Design review of the part built by this model. Coordinates are the model's own, in mm. Face numbers are marked on the shaded views. A direction names the side the tool comes from. Coordinates: 2 decimals unless noted, no trailing zeros. Loops run counter-clockwise (first coordinate to the right, second up) from the corner with the lowest first, then second, coordinate; pieces in that order, holes last. Notation, with made-up numbers: M 29,-29.75 L 50,-29.75 A26 cw 50,-1.75 Z; hole C 45.5,79 d11. An arc over 180 degrees is marked long. One line per item, written item: value.
```python
from build123d import *

# Parameters (mm, degrees)
SKETCH1_R           = 3
SKETCH1_R_2         = 1.6
BOSS_EXTRUDE1_DEPTH = 2
SKETCH1_3_R         = 1.6
BOSS_EXTRUDE2_DEPTH = 1
SKETCH5_R           = 1.5
BOSS_EXTRUDE3_DEPTH = 1
SKETCH6_R           = 2
BOSS_EXTRUDE4_DEPTH = 1
SKETCH8_R           = 1
BOSS_EXTRUDE5_DEPTH = 3


with BuildPart() as part:
    # Sketch1 → Boss-Extrude1 (new body)
    with BuildSketch(Plane(origin=(0, 0, 0), x_dir=(1, 0, 0), z_dir=(0, 1, 0))):
        with Locations((-0.522013312, 0.511138034)):
            Circle(SKETCH1_R)
        with Locations((-0.522013312, 0.511138034)):
            Circle(SKETCH1_R_2, mode=Mode.SUBTRACT)
    extrude(amount=BOSS_EXTRUDE1_DEPTH)

    # Sketch1<3> → Boss-Extrude2 (add)
    with BuildSketch(Plane(origin=(0, 0, 0), x_dir=(1, 0, 0), z_dir=(0, 1, 0))):
        with Locations((-0.522013312, 0.511138034)):
            Circle(SKETCH1_3_R)
    extrude(amount=BOSS_EXTRUDE2_DEPTH)

    # Sketch5 → Boss-Extrude3 (add)
    with BuildSketch(Plane.XZ):
        with Locations((-0.522013312, -0.511138034)):
            Circle(SKETCH5_R)
    extrude(amount=BOSS_EXTRUDE3_DEPTH)

    # Sketch6 → Boss-Extrude4 (add)
    with BuildSketch(Plane.XZ.offset(1)):
        with Locations((-0.522013312, -0.511138034)):
            Circle(SKETCH6_R)
    extrude(amount=BOSS_EXTRUDE4_DEPTH)

    # Sketch8 → Boss-Extrude5 (add)
    with BuildSketch(Plane(origin=(0, -2, 0), x_dir=(-1, 0, 0), z_dir=(0, -1, 0))):
        with Locations((0.522013312, 0.511138034)):
            Circle(SKETCH8_R)
    extrude(amount=BOSS_EXTRUDE5_DEPTH)


solid = part.part
```
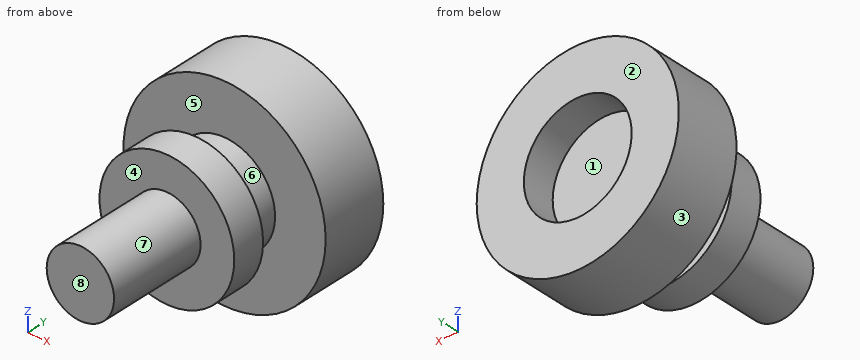
(1) We need section C-C on z = 0.8. State the section outline as (x, y) points (3 decimals), then the cut area to 3 significant figures.
Reply:
outline: M -3.22,0 L -1.251,0 L -1.251,-1 L -2.032,-1 L -2.032,-2 L 0.988,-2 L 0.988,-1 L 0.207,-1 L 0.207,0 L 2.176,0 L 2.176,2 L 0.395,2 L 0.395,1 L -1.439,1 L -1.439,2 L -3.22,2 Z
area: 13.4 mm2
(2) Mouldability with a two-part tool opening along Y and no side actions: class the marked faces 6, 7 and 8 as released by +Y, released by -Y, zero draft, split by the parting line, or undercut.
Reply:
face 6: undercut
face 7: zero draft
face 8: released by -Y
(3) To check wall thickness, follow line 1 along Y through (x, z) = (0.1, 1); line 2 along Y through (x, z) = (-0.55, 0.3); line 3 along Y through (x, z) = (1.4, 1.05). State the ranges of each line that lie inside material, in increasing order. Write a range as [from, to].
Reply:
line 1: y = [-2, -1], [0, 2]
line 2: y = [-5, 1]
line 3: y = [0, 2]
(4) Insertion check: pin 1 (1 mm diameter, centred on y = -3, z = 1.5, fed in from +X); pin 2 (3 mm diameter, centred on x = -0.52, z = -0.51, fed in from +Y); pin 3 (1.5 mm diameter, centred on y = -1, z = 1, fed in from -X). Each pin has a flat end and moves straight along its axis. Give the tip position at first contact, or say it passes through.
Reply:
pin 1: passes through
pin 2: stops at y = 1
pin 3: stops at x = -2.37
(5) We need section D-D on y = -1.25. State the section outline as (x, z) points.
Reply:
outline: C -0.52,-0.51 d4
(6) We need section A-A on z = -2.35. State the section outline as (x, y) points.
Reply:
outline: M -2.89,0 L 1.85,0 L 1.85,2 L -2.89,2 Z; M -1.31,-2 L 0.26,-2 L 0.26,-1 L -1.31,-1 Z
(7) We need section B-B on x = -0.9. State the section outline as (y, z) points.
Reply:
outline: M -5,-1.44 L -2,-1.44 L -2,-2.48 L -1,-2.48 L -1,-1.96 L 0,-1.96 L 0,-3.49 L 2,-3.49 L 2,-2.07 L 1,-2.07 L 1,1.04 L 2,1.04 L 2,2.46 L 0,2.46 L 0,0.94 L -1,0.94 L -1,1.45 L -2,1.45 L -2,0.41 L -5,0.41 Z
(8) Tool access review of the marked faces 1, 2, 3, 4 and 5: name each direction out of +Z, -Z, +X, -X, +Y, -Y from which nothing blocks a thin tool from reaching the whole face with its end or side.
Reply:
face 1: +Y
face 2: +Z, -Z, +X, -X, +Y
face 3: +Y, -Y
face 4: -Y
face 5: none
